from build123d import *

# Parameters (mm, degrees)
SKETCH1_R           = 100
BOSS_EXTRUDE1_DEPTH = 50
SKETCH2_W           = 100
SKETCH2_H           = 214.27053556
CUT_EXTRUDE1_DEPTH  = 45
SKETCH3_R           = 50
BOSS_EXTRUDE2_DEPTH = 20
SKETCH4_R           = 37.5
BOSS_EXTRUDE3_DEPTH = 10
CHAMFER1_SIZE       = 10
CHAMFER2_SIZE       = 7


with BuildPart() as part:
    # Sketch1 → Boss-Extrude1 (new body)
    with BuildSketch(Plane(origin=(0, 0, 0), x_dir=(1, 0, 0), z_dir=(0, 1, 0))):
        with Locations(Location((0, 0, 0), (0, 0, 270))):
            Circle(SKETCH1_R)
    extrude(amount=BOSS_EXTRUDE1_DEPTH)

    # Sketch2 → Cut-Extrude1 (cut)
    with BuildSketch(Plane(origin=(0, 50, 0), x_dir=(1, 0, 0), z_dir=(0, 1, 0))):
        Rectangle(SKETCH2_W, SKETCH2_H)
    extrude(amount=-CUT_EXTRUDE1_DEPTH, mode=Mode.SUBTRACT)

    # Sketch3 → Boss-Extrude2 (add)
    with BuildSketch(Plane(origin=(-50, 0, 0), x_dir=(0, 0, -1), z_dir=(1, 0, 0))):
        with Locations((0, 50)):
            Circle(SKETCH3_R)
    boss_extrude2 = extrude(amount=-BOSS_EXTRUDE2_DEPTH)

    # Mirror1: Boss-Extrude2 across plane
    add(boss_extrude2.mirror(Plane(origin=(0, 0, 0), x_dir=(0, 0, 1), z_dir=(1, 0, 0))))

    # Sketch4 → Boss-Extrude3 (add)
    with BuildSketch(Plane(origin=(70, 0, 0), x_dir=(0, 0, -1), z_dir=(1, 0, 0))):
        with Locations((0, 50)):
            Circle(SKETCH4_R)
    boss_extrude3 = extrude(amount=BOSS_EXTRUDE3_DEPTH)

    # Mirror2: Boss-Extrude3 across plane
    add(boss_extrude3.mirror(Plane(origin=(0, 0, 0), x_dir=(0, 0, 1), z_dir=(1, 0, 0))))

    # Chamfer1
    chamfer1_edges = [part.edges().sort_by_distance(p)[0] for p in [
        (100, 50, 0),
        (-100, 50, 0),
    ]]
    chamfer(chamfer1_edges, length=CHAMFER1_SIZE)

    # Chamfer2
    chamfer2_edges = [part.edges().sort_by_distance(p)[0] for p in [
        (-70, 100, 0),
        (70, 100, 0),
        (80, 87.5, 0),
        (-80, 87.5, 0),
    ]]
    chamfer(chamfer2_edges, length=CHAMFER2_SIZE)


solid = part.part
Could you check a few things on this model? Use its own coordinates, in mm. A direction names the side the tool comes from. Give positions to 0.01 mm unless a question says otherwise; leave off trailing zeros. Order: outer loops, then holes, each group sorted by start corner. A loop starts at its lowest first (then second) coordinate and runs counter-clockwise, first axis right, second up.
Item 1: If we section it at A-A, the plane z = 0: Write out the boundary of the cut face in (x, y).
Item 2: If we section it at D-D, the plane x = 39.5: Write out the boundary of the cut face in (y, z), plus the area to 3 significant figures.
Item 3: If we mould it in two halves opening along X, with no side actions, what happens to faces 1 (the face through (-70, 88, -3)), 2 (the face through (50, 43, 1)), 3 (the face through (79.66, 80.83, -0.68)), 4 (the face through (71.48, 87.49, -0.82))? For each: pulls with the +X half, pulls with the -X half, needs draft (parallel to the pull), parting line crosses it, or undercut.
Item 4: If we section it at C-C, the plane x = 0: Write out the boundary of the cut face in (y, z), plus the area to 3 significant figures.
Item 5: I'm going to push flat-ended pins straight in: pin 1 (21.5 mm diameter, centred on y = 64, z = 19, fed in from +X); pin 2 (8 mm diameter, centred on y = 40, z = 22, fed in from +X); pin 3 (6 mm diameter, centred on y = 49.5, z = -25.5, fed in from -X). Where does each tip first touch, or does it pass through?
Item 6: For faces 5 (the face through (-80, 62, 0)), 6 (the face through (-71.48, 87.49, -0.82)), 7 (the face through (80.5, 50, -5.9)), 8 (the face through (-1, 5, -1)), 9 (the face through (80, 62, 0)), which set-ups out of +Z, -Z, +X, -X, +Y, -Y let a thin tool reach every point of the face, with its end or its side?
Item 7: I need wall thicknesses on line 1 (X direction, y = 55.5, z = 19.5); line 2 (Y direction, x = 20.5, z = 80.5); line 3 (X direction, y = 26.5, z = 7). Which ranges of each line are inside material? Lowest first, please.
Item 8: If we section it at B-B, the plane y = 7.5: Write out the boundary of the cut face in (x, z).
Values:
1. outline: (-100, 0) - (100, 0) - (100, 40) - (90, 50) - (80, 50) - (80, 80.5) - (73, 87.5) - (70, 87.5) - (70, 93) - (63, 100) - (50, 100) - (50, 5) - (-50, 5) - (-50, 100) - (-63, 100) - (-70, 93) - (-70, 87.5) - (-73, 87.5) - (-80, 80.5) - (-80, 50) - (-90, 50) - (-100, 40) - close
2. outline: (0, -91.87) - (5, -91.87) - (5, 91.87) - (0, 91.87) - close
2. area: 919 mm2
3. face 1: pulls with the -X half
3. face 2: undercut
3. face 3: pulls with the +X half
3. face 4: needs draft
4. outline: (0, -100) - (5, -100) - (5, 100) - (0, 100) - close
4. area: 1,000 mm2
5. pin 1: stops at x = 80
5. pin 2: stops at x = 98.37
5. pin 3: stops at x = -90.07
6. face 5: +Z, -Z, -X, +Y
6. face 6: -X, +Y
6. face 7: +X, +Y
6. face 8: +Z, -Z, +Y
6. face 9: +Z, -Z, +X, +Y
7. line 1: x = -80 to -50, 50 to 80
7. line 2: y = 0 to 5
7. line 3: x = -99.75 to -50, 50 to 99.75
8. outline: (-50, -86.6) - (-50, 86.6) arc R100 ccw to start; (50, -86.6) arc R100 ccw to (50, 86.6) - close
